The listing builds one solid part. Answer for the finished solid, in the listing's coordinates (mm). A direction names the side the tool comes from. Round coordinates to 2 decimals unless told otherwise and drop trailing zeros. Order: outer loops, then holes, each group sorted by start corner. A loop starts at its lowest first (then second) coordinate and runs counter-clockwise, first axis right, second up. Notation, with made-up numbers: M 64.25,55 L 73.25,55 A3 ccw 73.25,59 Z; hole C 66.5,-27.75 d8. An arc over 180 degrees is marked long. Put each result on its own line as item: value. Start each with the question number.
1. The part is cut by section C-C (x = 49). Give the vertices of the cut face in (y, z), then the cut area to 3 significant figures.
2. The part is cut by section A-A (y = 16.5). Give the vertices of the cut face in (x, z), then the cut area to 3 significant figures.
3. Which of the six approach directions +Z, -Z, +X, -X, +Y, -Y give full straight-line access (tool end or side, diameter ignored) to faces 1 (the face through (5.56, 54.47, 7.58)), 2 (the face through (4.92, 55.09, -7.54)), 3 (the face through (6.459, 23.066, 3.915))?
4. The part is cut by section B-B (z = 5.5). Give the vertices of the cut face in (x, y), then the cut area to 3 significant figures.
5. Consider line 1 (Y direction, x = -2.5, z = 5.75); line 2 (Y direction, x = 40, z = 4); line 3 (X direction, y = 26, z = -4.75). Determine where each line is inside the solid, lowest interval first.
6. Each of these flat-tipped pins is pushed along its axis until it touches: pin 1 Ø1 at (x, z) = (33, -5) entering from +Y; pin 2 Ø3 at (y, z) = (61.5, 0) entering from -X; pin 3 Ø8 at (x, y) = (26, 45) entering from +Z; pin 4 Ø1.5 at (y, z) = (35.5, -3.5) entering from -X. Where does it stop, or does it pass through?
7. The part is cut by section D-D (z = -2.25). Give the vertices of the cut face in (x, y), then the cut area to 3 significant figures.
from build123d import *


with BuildPart() as part:
    # 扫描1: sweep along a path in 草图2
    with BuildLine(Plane.XY) as sweep_1_path:
        Line((0, 0), (0, 45.495221089))
        ThreePointArc((0, 45.495221089), (4.31309835, 55.907961623), (14.725838884, 60.221059973))
        Line((14.725838884, 60.221059973), (67.177001903, 60.221059973))
    # 草图3 → 扫描1 (sweep)
    with BuildSketch(Plane(origin=(0, 0, 0), x_dir=(1, 0, 0), z_dir=(0, 1, 0))):
        Polygon((4.259864643, -7.609541104), (8.719988229, -0.115619555), (4.460123586, 7.49392155), (-4.259864643, 7.609541104), (-8.719988229, 0.115619555), (-4.460123586, -7.49392155), align=None)
    sweep(path=sweep_1_path.line)


solid = part.part
Resolved:
1. outline: M 51.5,0.12 L 55.76,-7.49 L 64.48,-7.61 L 68.94,-0.12 L 64.68,7.49 L 55.96,7.61 Z
1. area: 198 mm2
2. outline: M -8.72,-0.12 L -4.26,-7.61 L 4.46,-7.49 L 8.72,0.12 L 4.26,7.61 L -4.46,7.49 Z
2. area: 198 mm2
3. face 1: +Z, -X, +Y
3. face 2: -Z, +X, -Y
3. face 3: +Z, +X, -Y
4. outline: M -5.58,0 L 5.52,0 L 5.52,45.5 A9.21 cw 14.73,54.71 L 67.18,54.71 L 67.18,65.8 L 14.73,65.8 A20.3 ccw -5.58,45.5 Z
4. area: 1,340 mm2
5. line 1: 0 to 55.97
5. line 2: 53.81 to 66.64
5. line 3: -5.96 to 6
6. pin 1: y = 66.33
6. pin 2: x = -3.69
6. pin 3: through
6. pin 4: x = -7.15
7. outline: M -7.45,0 L 7.4,0 L 7.4,45.5 A7.33 cw 14.73,52.83 L 67.18,52.83 L 67.18,67.67 L 14.73,67.67 A22.18 ccw -7.45,45.5 Z
7. area: 1,800 mm2
